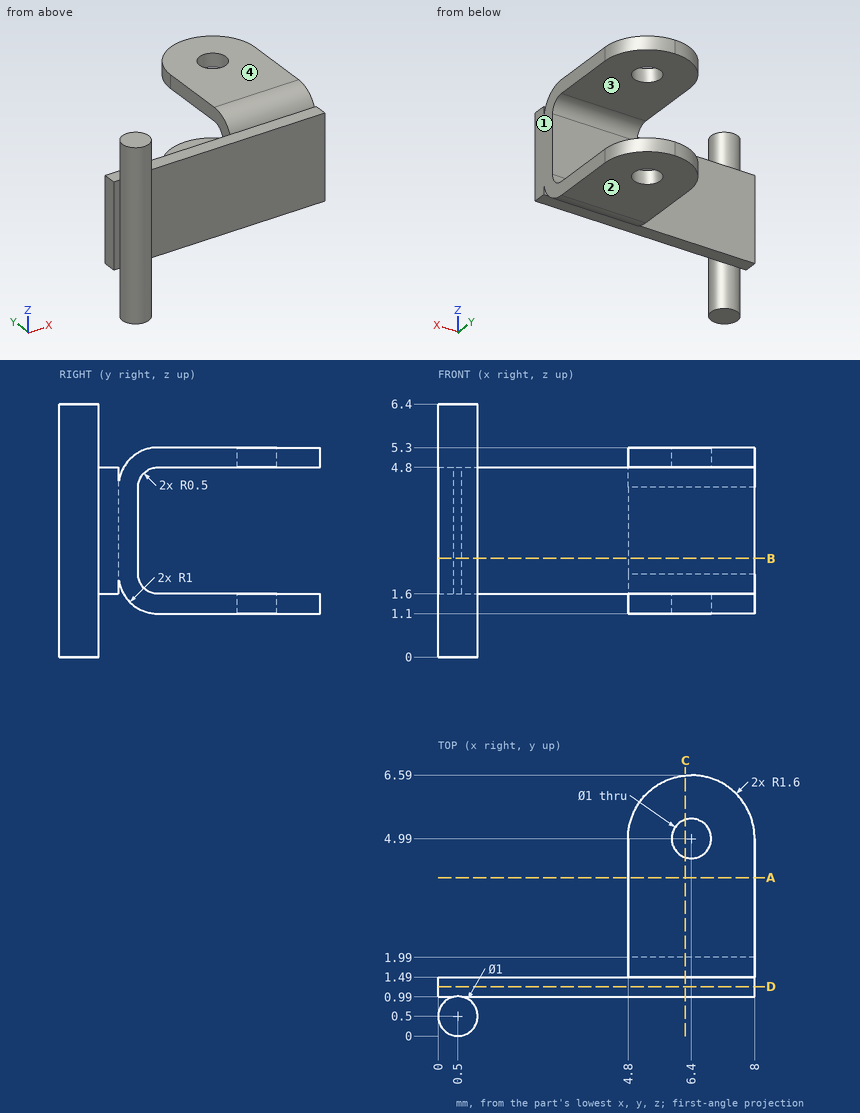
Geometry check sheet. Reference: drawing and pictorial views, mm from the part's lowest x, y, z. Coordinates: 2 decimals unless noted, no trailing zeros. Order: outer loops, then holes, each group sorted by start corner. A loop starts at its lowest first (then second) coordinate and runs counter-clockwise, first axis right, second up. Notation, with made-up numbers: M 48.25,2 L 100.25,2 A9 ccw 100.25,17 Z; hole C -15.75,56 d3. An arc over 180 degrees is marked long. Return JSON: item names as keys, results as strings.
1) Release check for a two-part mould opening along Z. For the marked faces 1, 2, 3 and 4 record: +Z half, -Z half, draft (parallel to the pull), parting line (faces both ways), or undercut.
Answer list:
{"face 1": "draft", "face 2": "-Z half", "face 3": "undercut", "face 4": "+Z half"}
2) Thickness scan on L1, parallel to Z at x = 5, y = 4; L2, parallel to Y at x = 7, z = 4.25; L3, parallel to Y at x = 2, z = 3.75. Record the ranges inside material, lowest first. Write a range as [from, to].
Answer list:
{"L1": "[1.1, 1.6], [4.8, 5.3]", "L2": "[0.99, 1.99]", "L3": "[0.99, 1.49]"}
3) Cross-section at D-D, the plane y = 1.25. Record the boundary of the cut face in (x, z).
Answer list:
{"outline": "M 0,1.6 L 8,1.6 L 8,4.8 L 0,4.8 Z"}
4) Cross-section at B-B, the plane z = 2.5. Record the boundary of the cut face in (x, y).
Answer list:
{"outline": "M 0,0.99 L 0.4,0.99 A0.5 ccw long 0.6,0.99 L 8,0.99 L 8,1.99 L 4.8,1.99 L 4.8,1.49 L 0,1.49 Z"}
5) Cross-section at A-A, the plane y = 4. Record the boundary of the cut face in (x, z), and give its area (3 significant figures).
Answer list:
{"outline": "M 4.8,1.1 L 8,1.1 L 8,1.6 L 4.8,1.6 Z; M 4.8,4.8 L 8,4.8 L 8,5.3 L 4.8,5.3 Z", "area": "3.20 mm2"}
6) Cross-section at C-C, the plane x = 6.25. Record the boundary of the cut face in (y, z).
Answer list:
{"outline": "M 0.99,1.6 L 1.49,1.6 L 1.49,2.1 A1 ccw 2.49,1.1 L 4.51,1.1 L 4.51,1.6 L 2.49,1.6 A0.5 cw 1.99,2.1 L 1.99,4.3 A0.5 cw 2.49,4.8 L 4.51,4.8 L 4.51,5.3 L 2.49,5.3 A1 ccw 1.49,4.3 L 1.49,4.8 L 0.99,4.8 Z; M 5.47,1.1 L 6.58,1.1 L 6.58,1.6 L 5.47,1.6 Z; M 5.47,4.8 L 6.58,4.8 L 6.58,5.3 L 5.47,5.3 Z"}
7) Gauge pin test, flat ends, axial feed: pin 1 (1.8 mm diameter, centred on x = 6, z = 3, fed in from +Y); pin 2 (0.6 mm diameter, centred on x = 2.5, y = 1.5, fed in from +Z); pin 3 (2.5 mm diameter, centred on x = 3.5, z = 3, fed in from -Y). Record the tip position at first contact, or that the pin passes through.
Answer list:
{"pin 1": "y = 1.99", "pin 2": "z = 4.8", "pin 3": "y = 0.99"}
